Can you work these out from the drawing? Everything is in mm from the part's minimum corner. A direction names the side the tool comes from. Coordinates: 2 decimals unless noted, no trailing zeros. Order: outer loops, then holes, each group sorted by start corner. A loop starts at its lowest first (then second) coordinate and runs counter-clockwise, first axis right, second up. Notation, with made-up numbers: M 70,-19 L 84,-19 A13 ccw 84,2 Z; hole C -8.75,-28 d3. An arc over 180 degrees is marked long. Answer as CSV lines item,"result". Start each with the question number.
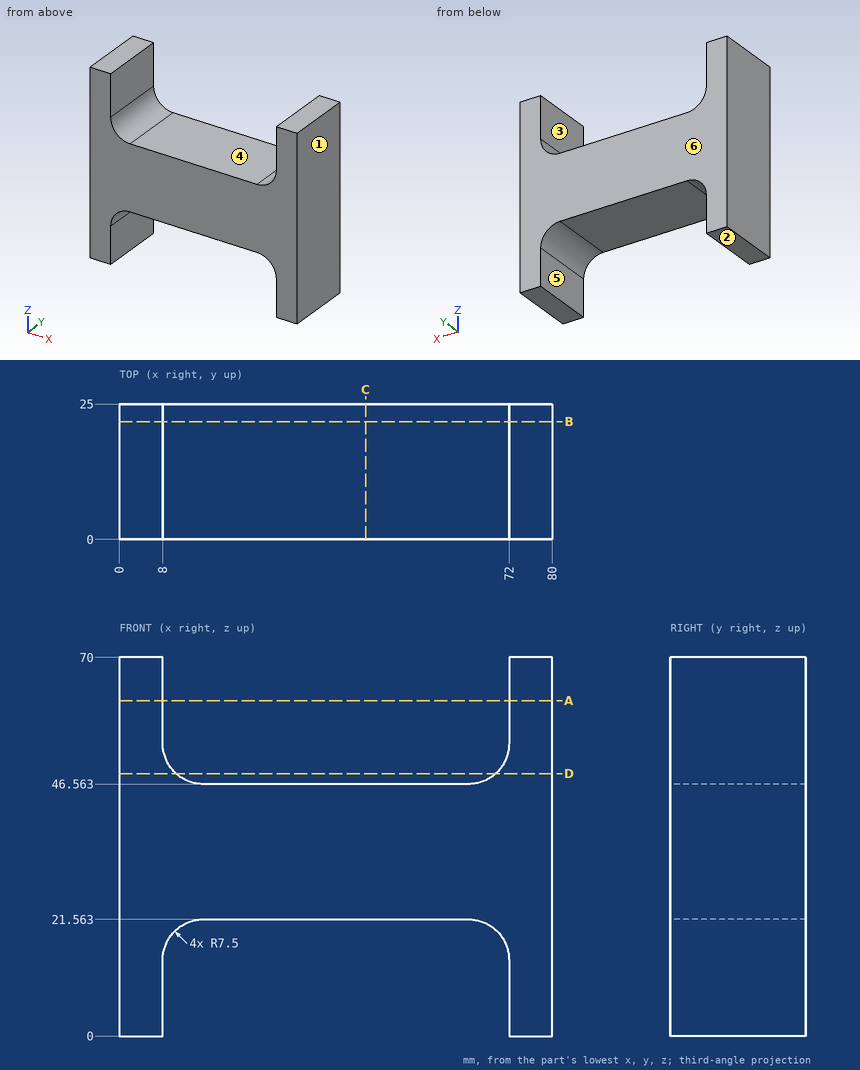
1) Suppose I cut it at C-C on x = 45.5. Please give me the cut outline in (y, z), plus the area to 3 significant figures.
2) I need wall thicknesses on line 1 (X direction, y = 6, z = 9); line 2 (Z direction, x = 31.5, y = 23.75); line 3 (X direction, y = 6.75, z = 49.5). Which ranges of each line are inside material? Lowest first, please. Write a range as [from, to].
3) Which directions (+Z, -Z, +X, -X, +Y, -Y) give clear straight access to the entire face, cutting with the end or side of a thin tool? Please do the marked faces 4, 5 and 6.
4) Suppose I cut it at A-A on z = 62. Please give me the cut outline in (x, y).
5) Will these pins go through, and if not, where does the flat tip stop? pin 1 Ø7.5 at (x, y) = (45, 13) entering from -Z; pin 2 Ø1.5 at (x, y) = (26, 10) entering from +Z.
6) If we mould it in two halves opening along X, with no side actions, what happens to the marked faces 1, 2 and 3? For each: released by +X, released by -X, zero draft, split by the parting line, or undercut.
7) Suppose I cut it at D-D on z = 48.5. Please give me the cut outline in (x, y), plus the area to 4 significant figures.
8) Suppose I cut it at B-B on y = 21.75. Please give me the cut outline in (x, z), plus the area to 3 significant figures.
Output:
1,outline,"M 0,21.56 L 25,21.56 L 25,46.56 L 0,46.56 Z"
1,area,"625 mm²"
2,line 1,"[0, 8], [72, 80]"
2,line 2,"[21.56, 46.56]"
2,line 3,"[0, 9.55], [70.45, 80]"
3,face 4,"+Z, +Y, -Y"
3,face 5,"-Z, +Y, -Y"
3,face 6,"+Z, -Z, +X, -X, +Y"
4,outline,"M 0,0 L 8,0 L 8,25 L 0,25 Z; M 72,0 L 80,0 L 80,25 L 72,25 Z"
5,pin 1,"z = 21.56"
5,pin 2,"z = 46.56"
6,face 1,"released by +X"
6,face 2,"zero draft"
6,face 3,"undercut"
7,outline,"M 0,0 L 10.47,0 L 10.47,25 L 0,25 Z; M 69.53,0 L 80,0 L 80,25 L 69.53,25 Z"
7,area,"523.5 mm²"
8,outline,"M 0,0 L 8,0 L 8,14.06 A7.5 cw 15.5,21.56 L 64.5,21.56 A7.5 cw 72,14.06 L 72,0 L 80,0 L 80,70 L 72,70 L 72,54.06 A7.5 cw 64.5,46.56 L 15.5,46.56 A7.5 cw 8,54.06 L 8,70 L 0,70 Z"
8,area,"2,770 mm²"
